Check sheet for the modelled part. Datum: model origin and axes. Units: mm. Face numbers are marked on the shaded views. A direction names the side the tool comes from. Round coordinates to 2 decimals unless told otherwise and drop trailing zeros. Loops run counter-clockwise (first coordinate to the right, second up) from the corner with the lowest first, then second, coordinate; pieces in that order, holes last. Notation, with made-up numbers: M 12.5,15.5 L 64.5,15.5 A18 cw 64.5,19.5 Z; hole C 61.25,54 d6. An arc over 180 degrees is marked long. Write item = value, one per line. Start each with the question number.
(1) Mould release check, pull along Y, two halves, no side actions. Record for the marked faces 1, 2, 3 and 4: pulls with the +Y half, pulls with the -Y half, needs draft (parallel to the pull), parting line crosses it, or undercut.
(2) Cross-section at C-C on z = -3.75. Record the boundary of the cut face in (x, y).
(3) Scan lines: L1, parallel to Y at x = 5, z = -3.4; L2, parallel to Y at x = 5, z = 0.6; L3, parallel to Y at x = 5.75, z = 1.25. Record each from-to range of solid material in increasing order. Write a range as from..to.
(4) Set-up check for the marked faces 5 and 6: record each of +Z, -Z, +X, -X, +Y, -Y from which the full face is reachable in a straight line by a thin tool's end or side.
(5) Cross-section at B-B on x = 5. Record the boundary of the cut face in (y, z).
(6) Cross-section at A-A on y = 11.5. Record the boundary of the cut face in (x, z).
(7) Cross-section at D-D on y = 1.5. Record the boundary of the cut face in (x, z).
(8) Go/stop test with flat-tipped pins: P1, Ø2, axis at x = 5.5, z = -2.5, coming from the +Y side; P2, Ø1.5, axis at y = 10.5, z = -3.5, coming from the +X side; P3, Ø1, axis at y = 10.5, z = -3, coming from the +X side. Record where each tip stops, or that it passes through.
Autodesk Inventor part; units mm, degrees
ref_plane "XZ Plane" through (0, 0, 0) normal (0, 1, 0) x (-1, 0, 0)
ref_plane "XY Plane" through (0, 0, 0) normal (0, 0, 1) x (1, 0, 0)
ref_plane "Arbeitsebene1" through (5, 7.0959, 0) normal (1, 0, 0) x (0, 1, 0)
sketch "Skizze1" plane through (5, 7.0959, 0) normal (1, 0, 0) x (0, 1, 0)
  arc A0 (6.9041, 0) -> (9.9041, 3) centre (6.9041, 3) ccw
  line L0 (6.9041, 0) -> (-7.0959, 0)
  arc A1 (-10.0959, 3) -> (-7.0959, 0) centre (-7.0959, 3) ccw
  line L1 (9.6536, 1.8) -> (-9.8455, 1.8)
  dimension "d0" = 1.8
extrude "Extrusion1" add sketch "Skizze1" along normal mid plane 10
ref_plane "Arbeitsebene2" through (5, -12.9041, -4.7) normal (0, 0, -1) x (-1, 0, 0)
sketch "Skizze2" plane through (5, -12.9041, -4.7) normal (0, 0, -1) x (-1, 0, 0)
  arc A0 (-2.8982, 26.7749) -> (2.8982, 26.7749) centre (0, 26) ccw
  arc A1 (2.7927, 12.9041) -> (-2.7927, 12.9041) centre (0, 14) ccw
  circle A2 centre (0, 14) radius 3
  circle A3 centre (0, 26) radius 3
  circle A4 centre (0, 26) radius 2
  circle A5 centre (0, 14) radius 2
  point P0 (5, 12.9041)
  dimension "d3" = 0
  dimension "d4" = 4
extrude "Extrusion2" add sketch "Skizze2" against normal up to surface (6.5 mm away)
sketch "Skizze3" plane through (5, 13.0959, -4.7) normal (0, 0, -1) x (-1, 0, 0)
  circle A0 centre (0, 0) radius 2
  circle A1 centre (0, -12) radius 2
  point P0 (5, -13.0959)
extrude "Extrusion3" cut sketch "Skizze3" against normal up to surface (6.5 mm away)
sketch "Skizze4" plane through (0, -2.7495, 1.8) normal (0, 0, 1) x (1, 0, 0)
  circle A0 centre (5, 15.8455) radius 2
  circle A1 centre (5, 3.8455) radius 2
  line L0 (0, 0) -> (10, 0)
  line L1 (10, 19.4991) -> (10, 0)
  line L2 (0, 19.4991) -> (10, 19.4991)
  line L3 (0, 0) -> (0, 19.4991)
  circle A2 centre (5, 15.8455) radius 2
  line L4 (7.8866, 15.8762) -> (6.4699, 13.361)
  line L5 (6.4699, 13.361) -> (3.5833, 13.3303)
  line L6 (3.5833, 13.3303) -> (2.1134, 15.8148)
  line L7 (2.1134, 15.8148) -> (3.5301, 18.33)
  line L8 (3.5301, 18.33) -> (6.4167, 18.3607)
  line L9 (6.4167, 18.3607) -> (7.8866, 15.8762)
  line L10 (7.8866, 3.8762) -> (6.4699, 1.361)
  line L11 (6.4699, 1.361) -> (3.5833, 1.3303)
  line L12 (3.5833, 1.3303) -> (2.1134, 3.8148)
  line L13 (2.1134, 3.8148) -> (3.5301, 6.33)
  line L14 (3.5301, 6.33) -> (6.4167, 6.3607)
  line L15 (6.4167, 6.3607) -> (7.8866, 3.8762)
  point P0 (0, 2.7495)
  dimension "d9" = 5
extrude "Extrusion4" cut sketch "Skizze4" against normal blind 1 contours L4 L5 L6 L7 L8 L9 | L10 L11 L12 L13 L14 L15
properties part number "Isolationsmasse"
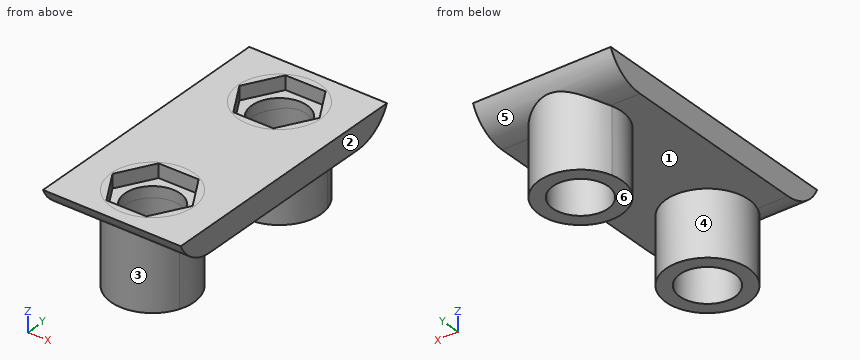
Result:
q1.face_1 = undercut
q1.face_2 = needs draft
q1.face_3 = pulls with the -Y half
q1.face_4 = undercut
q2.outline = M 2.1,13.87 A3 ccw long 7.9,13.87 A3 ccw Z; M 2.21,0 A3 ccw 7.79,0 A3 ccw long Z; hole C 5,1.1 d4; hole C 5,13.1 d4
q3.L1 = -1.9..-0.9, 3.1..4.1, 10.1..11.1, 15.1..16.1
q3.L2 = -1.9..-0.9, 3.1..11.1, 15.1..16.1
q3.L3 = -2.44..-1.4, 3.6..10.6, 15.6..16.44
q4.face_5 = -Z, +Y
q4.face_6 = -Z, +X, -X, +Y, -Y
q5.outline = M -2.75,1.8 A3 ccw -1.9,0.68 L -1.9,-4.7 L -0.9,-4.7 L -0.9,0.8 L -1.4,0.8 L -1.4,1.8 Z; M 3.1,-4.7 L 4.1,-4.7 L 4.1,0 L 10.1,0 L 10.1,-4.7 L 11.1,-4.7 L 11.1,0.8 L 10.6,0.8 L 10.6,1.8 L 3.6,1.8 L 3.6,0.8 L 3.1,0.8 Z; M 15.1,-4.7 L 16.1,-4.7 L 16.1,0.85 A3 ccw 16.75,1.8 L 15.6,1.8 L 15.6,0.8 L 15.1,0.8 Z
q6.outline = M 0,0 L 2.46,0 L 2.46,-4.7 L 3.79,-4.7 L 3.79,0.8 L 3.04,0.8 L 3.04,1.8 L 0,1.8 Z; M 6.21,-4.7 L 7.54,-4.7 L 7.54,0 L 10,0 L 10,1.8 L 6.97,1.8 L 6.97,0.8 L 6.21,0.8 Z
q7.outline = M 0,0 L 2.03,0 L 2.03,-4.7 L 3.04,-4.7 L 3.04,0.8 L 2.36,0.8 L 2.36,1.8 L 0,1.8 Z; M 6.96,-4.7 L 7.97,-4.7 L 7.97,0 L 10,0 L 10,1.8 L 7.67,1.8 L 7.67,0.8 L 6.96,0.8 Z
q8.P1 = 16.1
q8.P2 = 7.36
q8.P3 = 7.15
